from build123d import *

# Parameters (mm, degrees)
F1_DEPTH  = 25.4
F3_DEPTH  = 38.1
F2_W      = 38.1
F2_H      = 12.7
F4_DEPTH  = 38.1
F6_DEPTH  = 12.7
F7_R      = 12.7
F8_DEPTH  = 38.1
F10_DEPTH = 12.7
F12_DEPTH = 38.1


with BuildPart() as f1:
    # F0 (on Top) → F1 (new body)
    with BuildSketch(Plane.XY):
        with BuildLine():
            Line((23.2921783298, 36.4497782979), (-65.6065904021, 36.9176649997))
            Line((-65.6065904021, 36.9176649997), (-65.6065904021, 24.2176649997))
            ThreePointArc((-65.6065904021, 24.2176649997), (-56.626334281, 20.4979211207), (-52.9065904021, 11.5176649997))
            ThreePointArc((-52.9065904021, 11.5176649997), (-56.626334281, 2.5374088786), (-65.6065904021, -1.1823350003))
            Line((-65.6065904021, -1.1823350003), (-65.6065904021, -13.8823350003))
            Line((-65.6065904021, -13.8823350003), (23.2921783298, -13.8823350003))
            Line((23.2921783298, -13.8823350003), (23.2921783298, 36.4497782979))
        make_face()
        with BuildLine():
            Line((-65.6065904021, 24.2176649997), (-65.6065904021, 36.9176649997))
            ThreePointArc((-65.6065904021, 36.9176649997), (-91.0065904021, 11.5176649997), (-65.6065904021, -13.8823350003))
            Line((-65.6065904021, -13.8823350003), (-65.6065904021, -1.1823350003))
            ThreePointArc((-65.6065904021, -1.1823350003), (-78.3065904021, 11.5176649997), (-65.6065904021, 24.2176649997))
        make_face()
    extrude(amount=F1_DEPTH)

    # F2 (on face) → F3 (join)
    with BuildSketch(Plane.XY.offset(25.4)):
        Polygon((-14.8078216702, 36.9176649997), (-14.8078216702, 36.6503039473), (23.2921783298, 36.4497782979), (23.2921783298, 36.9176649997), align=None)
        Polygon((-14.8078216702, 24.2176649997), (23.2921783298, 24.2176649997), (23.2921783298, 36.4497782979), (-14.8078216702, 36.6503039473), align=None)
    extrude(amount=F3_DEPTH)

    # F2 (on face) → F4 (join)
    with BuildSketch(Plane.XY.offset(25.4)):
        with Locations((4.2421783298, -7.5323350003)):
            Rectangle(F2_W, F2_H)
    extrude(amount=F4_DEPTH)

    # F5 (on face) → F6 (join)
    with BuildSketch(Plane(origin=(0, 36.9176649997, 0), x_dir=(-1, 0, 0), z_dir=(0, 1, 0))):
        with BuildLine():
            Line((-23.2594181519, 63.5), (14.7750614924, 63.5))
            ThreePointArc((14.7750614924, 63.5), (-4.2421783298, 82.5172398221), (-23.2594181519, 63.5))
        make_face()
    extrude(amount=-F6_DEPTH)

    # F7 (on face) → F8 (cut)
    with BuildSketch(Plane(origin=(0, 36.9176649997, 0), x_dir=(-1, 0, 0), z_dir=(0, 1, 0))):
        with Locations((-4.2421783298, 63.5)):
            Circle(F7_R)
    extrude(amount=-F8_DEPTH, mode=Mode.SUBTRACT)

    # F9 (on face) → F10 (join)
    with BuildSketch(Plane.XZ.offset(13.8823350003)):
        with BuildLine():
            Line((-14.8078216702, 63.5), (23.2921783298, 63.5))
            ThreePointArc((23.2921783298, 63.5), (4.2421783298, 82.55), (-14.8078216702, 63.5))
        make_face()
    extrude(amount=-F10_DEPTH)

    # F11 (on face) → F12 (cut)
    with BuildSketch(Plane.XZ.offset(13.8823350003)):
        with BuildLine():
            ThreePointArc((-8.4578216702, 63.5), (4.2421783298, 50.8), (16.9421783298, 63.5))
            Line((16.9421783298, 63.5), (-8.4578216702, 63.5))
        make_face()
        with BuildLine():
            Line((-8.4578216702, 63.5), (16.9421783298, 63.5))
            ThreePointArc((16.9421783298, 63.5), (4.2421783298, 76.2), (-8.4578216702, 63.5))
        make_face()
    extrude(amount=-F12_DEPTH, mode=Mode.SUBTRACT)


solid = f1.part
Geometry: final body of the model. Coordinates: model frame, mm. A direction names the side the tool comes from. Round coordinates to 2 decimals unless told otherwise and drop trailing zeros. Order: outer loops, then holes, each group sorted by start corner. A loop starts at its lowest first (then second) coordinate and runs counter-clockwise, first axis right, second up. Notation, with made-up numbers: (29, 79) -> (81, 79) arc R15 cw to (81, 96) -> close; hole circle Ø3 at (-21.75, 26.5). An arc over 180 degrees is marked (long way). Put each result on its own line as item: value. Start each with the question number.
Q1. Reachability of faces 5 (the flat face through (4, 24.218, 47)), 6 (the cylindrical face through (4.661, -7.621, 82.545)), 7 (the flat face through (-14.808, -8, 44)) from +Z, -Z, +X, -X, +Y, -Y: full face, straight path, thin tool, end or side. Return the list, or none.
Q2. Section A-A on y = 2. Return the cut outline in (x, z), and give its area (3 significant figures).
Q3. Section D-D on y = -7. Return the cut outline in (x, z).
Q4. First-contact query: pin 1 (14 mm diameter, centred on y = -4.5, z = 50, fed in from -X); pin 2 (4 mm diameter, centred on x = -77, z = 27, fed in from -Y); pin 3 (6 mm diameter, centred on x = -40.5, z = 30, fed in from -Y); pin 4 (2 mm diameter, centred on x = 11, y = 17, fed in from +Z). Flat tips, straight axial feed; report the tip coordinate or a pass-through.
Q5. Line query: probe 1 along X at (y, z) = (32, 63); probe 2 along Y at (x, z) = (-66, 16); probe 3 along Z at (x, y) = (-4, 18). Output: solid intervals per line, ascending.
Q6. Section B-B on z = 67.5. Return the cut outline in (x, y), and give its area (3 significant figures).
Q7. Pull-direction query (X, two-part tool) for faces 1 (the cylindrical face through (3.824, 30.657, 82.513)), 2 (the flat face through (4, -1.182, 48)), 3 (the cylindrical face through (5.9, 30.66, 76.09)), 4 (the cylindrical face through (16.356, -7.621, 67.315)); classes: +X half, -X half, draft (parallel to the pull), parting line (faces both ways), or undercut.
Q8. Section C-C on x = 0.5. Return the cut outline in (y, z), and give its area (3 significant figures).
Ans:
1. face 5: +Z, +X, -X
1. face 6: +Z, +Y, -Y
1. face 7: +Z, -X, +Y, -Y
2. outline: (-89.16, 0) -> (-74.02, 0) -> (-74.02, 25.4) -> (-89.16, 25.4) -> close; (-57.2, 0) -> (23.29, 0) -> (23.29, 25.4) -> (-57.2, 25.4) -> close
2. area: 2,430 mm2
3. outline: (-82.99, 0) -> (23.29, 0) -> (23.29, 63.5) arc R19.05 ccw to (-14.81, 63.5) -> (-14.81, 25.4) -> (-82.99, 25.4) -> close; hole circle Ø25.4 at (4.24, 63.5)
4. pin 1: stops at x = -14.81
4. pin 2: stops at y = -11.75
4. pin 3: passes through
4. pin 4: stops at z = 25.4
5. probe 1: x = -14.81 to -8.45, 16.93 to 23.29
5. probe 2: y = -13.88 to -1.18, 24.21 to 36.91
5. probe 3: z = 0 to 25.4
6. outline: (-14.38, -13.88) -> (-7.81, -13.88) -> (-7.81, -1.18) -> (-14.38, -1.18) -> close; (-14.35, 24.22) -> (-7.81, 24.22) -> (-7.81, 36.92) -> (-14.35, 36.92) -> close; (16.3, -13.88) -> (22.87, -13.88) -> (22.87, -1.18) -> (16.3, -1.18) -> close; (16.3, 24.22) -> (22.83, 24.22) -> (22.83, 36.92) -> (16.3, 36.92) -> close
6. area: 333 mm2
7. face 1: parting line
7. face 2: draft
7. face 3: undercut
7. face 4: undercut
8. outline: (-13.88, 0) -> (36.57, 0) -> (36.57, 25.4) -> (36.92, 25.4) -> (36.92, 51.36) -> (24.22, 51.36) -> (24.22, 25.4) -> (-1.18, 25.4) -> (-1.18, 51.36) -> (-13.88, 51.36) -> close; (-13.88, 75.64) -> (-1.18, 75.64) -> (-1.18, 82.18) -> (-13.88, 82.18) -> close; (24.22, 75.64) -> (36.92, 75.64) -> (36.92, 82.15) -> (24.22, 82.15) -> close
8. area: 2,110 mm2
